Part model, mm, in its own coordinate system. A direction names the side the tool comes from. Give positions to 0.01 mm unless a question says otherwise; leave off trailing zeros. Order: outer loops, then holes, each group sorted by start corner. A loop starts at its lowest first (then second) coordinate and runs counter-clockwise, first axis right, second up. Notation, with made-up numbers: M 67.5,74.25 L 83.5,74.25 A31 ccw 83.5,106.25 Z; hole C -15.5,25.25 d5. An arc over 180 degrees is marked long. Return JSON: item names as keys, results as strings.
Autodesk Inventor part; units mm, degrees
ref_plane "YZ Plane" through (0, 0, 0) normal (1, 0, 0) x (0, 1, 0)
ref_plane "XZ Plane" through (0, 0, 0) normal (0, 1, 0) x (-1, 0, 0)
ref_plane "XY Plane" through (0, 0, 0) normal (0, 0, 1) x (1, 0, 0)
sketch "Skizze2" plane through (0, 0, 0) normal (0, 0, 1) x (1, 0, 0)
  line L0 (-20, -10) -> (20, -10)
  line L1 (20, -10) -> (20, 10)
  line L2 (20, 10) -> (-20, 10)
  line L3 (-20, 10) -> (-20, -10)
  line L4 (-20, -10) -> (20, 10) construction
  line L5 (20, -10) -> (-20, 10) construction
  point P0 (0, 0)
  dimension "d0" = 40
  dimension "d1" = 20
extrude "Extrusion1" add sketch "Skizze2" along normal blind 35
sketch "Skizze3" plane through (0, 0, 0) normal (0, 0, -1) x (-1, 0, 0)
  circle A0 centre (0, 0) radius 25
  dimension "d4" = 50
extrude "Extrusion2" add sketch "Skizze3" along normal blind 10
sketch "Skizze4" plane through (0, 0, -10) normal (0, 0, -1) x (-1, 0, 0)
  line L0 (10, -20) -> (-10, -20)
  line L1 (-20, -10) -> (-20, 10)
  line L2 (-10, 20) -> (10, 20)
  line L3 (20, 10) -> (20, -10)
  line L4 (20, -20) -> (-20, 20) construction
  line L5 (-20, -20) -> (20, 20) construction
  arc A0 (-20, -10) -> (-10, -20) centre (-10, -10) ccw
  arc A1 (-10, 20) -> (-20, 10) centre (-10, 10) ccw
  arc A2 (20, 10) -> (10, 20) centre (10, 10) ccw
  arc A3 (10, -20) -> (20, -10) centre (10, -10) ccw
  point P0 (0, 0)
  dimension "d7" = 40
  dimension "d8" = 40
  dimension "d9" = 10
extrude "Extrusion3" add sketch "Skizze4" along normal blind 100
sketch "Skizze5" plane through (0, 0, -110) normal (0, 0, -1) x (-1, 0, 0)
  circle A0 centre (0, 0) radius 10
  dimension "d12" = 20
extrude "Extrusion4" cut sketch "Skizze5" against normal up to surface (100 mm away)
fillet "Rundung1" radius 2 9 edges at (17.0711, -17.0711, -110) (0, -20, -110) (-17.0711, -17.0711, -110) (-20, 0, -110) (-17.0711, 17.0711, -110) (0, 20, -110) (17.0711, 17.0711, -110) (20, 0, -110) (10, 0, -110)
properties part number "Hubvorrichtung"
Q1. 3-axis set-ups, long thin cutter, end or side, ignore diameter. For faces 5 (the flat face through (20, 0, -58)), 6 (the cylindrical face through (-17.15, -16.99, -58.31)), 7 (the cylindrical face through (17.15, 16.99, -58.31)), 8 (the flat face through (-20.3, -1.7, -10)), 9 (the flat face through (-20, 0, -58)): which of +Z, -Z, +X, -X, +Y, -Y reach the whole face in a straight line?
Established:
{"face 5": "-Z, +X, +Y, -Y", "face 6": "-Z, -X, -Y", "face 7": "-Z, +X, +Y", "face 8": "-Z", "face 9": "-Z, -X, +Y, -Y"}
Q2. Pin check, flat tips, straight feed: pin 1 (6 mm diameter, centred on y = 0.5, z = 13.5, fed in from -X); pin 2 (6 mm diameter, centred on x = -0.5, z = -35, fed in from +Y); pin 3 (1.5 mm diameter, centred on x = -13.5, z = -87, fed in from -Y). Stop position of each tip, or through.
Established:
{"pin 1": "stops at x = -20", "pin 2": "stops at y = 20", "pin 3": "stops at y = -19.61"}
Q3. Band-saw the part on C-C (y = 0). Give the cut face in (x, z), then the cut area to 3 significant figures.
Established:
{"outline": "M -25,-10 L -20,-10 L -20,-108 A2 ccw -18,-110 L -12,-110 A2 ccw -10,-108 L -10,-10 L 10,-10 L 10,-108 A2 ccw 12,-110 L 18,-110 A2 ccw 20,-108 L 20,-10 L 25,-10 L 25,0 L 20,0 L 20,35 L -20,35 L -20,0 L -25,0 Z", "area": "3,900 mm²"}
Q4. Two-plate mould, pull along X, no slides. Class faces 1 (the flat face through (0, 20, -58)), 2 (the flat face through (0, 0, -10)), 3 (the cylindrical face through (-23.846, -7.509, -4.93)), 4 (the cylindrical face through (2.17, -9.76, -59.69)): +X half, -X half, draft (parallel to the pull), parting line (faces both ways), or undercut.
Established:
{"face 1": "draft", "face 2": "undercut", "face 3": "parting line", "face 4": "undercut"}
Q5. Band-saw the part on A-A (z = -15.5). Give the cut face in (x, y), then the cut area to 3 significant figures.
Established:
{"outline": "M -20,-10 A10 ccw -10,-20 L 10,-20 A10 ccw 20,-10 L 20,10 A10 ccw 10,20 L -10,20 A10 ccw -20,10 Z; hole C 0,0 d20", "area": "1,200 mm²"}
Q6. Probe line 1 along Y through (x, z) = (0, -54); line 2 along X through (y, z) = (8, 25); line 3 along Z through (x, y) = (10.5, -15). List the from-to ranges inside material, lowest first.
Established:
{"line 1": "y = -20 to -10, 10 to 20", "line 2": "x = -20 to 20", "line 3": "z = -110 to 0"}
Q7. Band-saw the part on B-B (x = 0). Give the cut face in (y, z), then the cut area to 3 significant figures.
Established:
{"outline": "M -25,-10 L -20,-10 L -20,-108 A2 ccw -18,-110 L -12,-110 A2 ccw -10,-108 L -10,-10 L 10,-10 L 10,-108 A2 ccw 12,-110 L 18,-110 A2 ccw 20,-108 L 20,-10 L 25,-10 L 25,0 L 10,0 L 10,35 L -10,35 L -10,0 L -25,0 Z", "area": "3,200 mm²"}
